```python
from build123d import *
from build123d.topology import SkipClean

# Parameters (mm, degrees)
BOSS_EXTRUDE1_DEPTH = 1.5
SKETCH3_R           = 3.75
CUT_EXTRUDE1_DEPTH  = 0.9
SKETCH4_R           = 2.2
CUT_EXTRUDE2_DEPTH  = 0.9
SKETCH5_R           = 1.5
CUT_EXTRUDE3_DEPTH  = 6
CUT_EXTRUDE4_DEPTH  = 0.3


with BuildPart() as part:
    # Sketch1 → Boss-Extrude1 (new body)
    with BuildSketch(Plane(origin=(0, 0, 0), x_dir=(1, 0, 0), z_dir=(0, 1, 0))):
        Polygon((-13.430051813, 17.5), (-13.430051813, 0), (-11.430051813, 0), (-11.430051813, -2.5), (8.569948187, -2.5), (8.569948187, 0), (10.569948187, 0), (10.569948187, 17.5), align=None)
    extrude(amount=BOSS_EXTRUDE1_DEPTH)

    # Sketch3 → Cut-Extrude1 (cut)
    with BuildSketch(Plane.XZ):
        with Locations(Location((-1.430051813, -7.5, 0), (0, 0, 270))):
            Circle(SKETCH3_R)
    extrude(amount=-CUT_EXTRUDE1_DEPTH, mode=Mode.SUBTRACT)

    # Sketch4 → Cut-Extrude2 (cut)
    with BuildSketch(Plane.XZ.offset(-0.9)):
        with Locations(Location((-1.430051813, -7.5, 0), (0, 0, 270))):
            Circle(SKETCH4_R)
    extrude(amount=-CUT_EXTRUDE2_DEPTH, mode=Mode.SUBTRACT)

    # Sketch5 → Cut-Extrude3 (cut)
    with BuildSketch(Plane.XZ):
        with Locations(Location((-8.430051813, -13.5, 0), (0, 0, 270))):
            Circle(SKETCH5_R)
        with Locations(Location((5.569948187, -13.5, 0), (0, 0, 270))):
            Circle(SKETCH5_R)
    extrude(amount=-CUT_EXTRUDE3_DEPTH, mode=Mode.SUBTRACT)

    # Sketch6 → Cut-Extrude4 (cut)
    with SkipClean():  # the faces are left unmerged after this step: merging them gives an invalid solid
        with BuildSketch(Plane.XZ.offset(-0.9)):
            with BuildLine():
                Line((1.606805114, -9.7), (-4.466908741, -9.7))
                ThreePointArc((-4.466908741, -9.7), (-5.180051813, -7.5), (-4.466908741, -5.3))
                Line((-4.466908741, -5.3), (1.606805114, -5.3))
                ThreePointArc((1.606805114, -5.3), (2.319948187, -7.5), (1.606805114, -9.7))
            make_face()
        extrude(amount=-CUT_EXTRUDE4_DEPTH, mode=Mode.SUBTRACT)


solid = part.part
```
The model under review builds one solid part; all positions refer to its coordinate system, in mm. A direction names the side the tool comes from. Round coordinates to 2 decimals unless told otherwise and drop trailing zeros. Loops run counter-clockwise (first coordinate to the right, second up) from the corner with the lowest first, then second, coordinate; pieces in that order, holes last. Notation, with made-up numbers: (9, 51.25) -> (53, 51.25) arc R24 ccw to (53, 63.25) -> close; hole circle Ø2 at (-31, 73). An arc over 180 degrees is marked (long way). Answer as a JSON object with one key per item and string values. Group by question number.
1) Mouldability with a two-part tool opening along X and no side actions: class faces 5 (the face through (-2, 0, -12)), 6 (the face through (-4, 1.2, -7)), 7 (the face through (8.57, 1, 1)) as released by +X, released by -X, zero draft, split by the parting line, or undercut.
2) For line 1 (X direction, y = 0.7, z = -13.5); line 2 (X direction, y = 1.35, z = -7.5); line 3 (Z direction, x = -4.5, y = 0.3), list the stretches that pass through material, from the lowest coordinate up. Write a range as [from, to].
3) For faces 1 (the face through (10, 1, 0)), 2 (the face through (-1, 0.9, -5)), 3 (the face through (-12, 1, 0)), 4 (the face through (5.6, 0.7, -12)), list the 3-axis set-ups (+Z, -Z, +X, -X, +Y, -Y) from which the entire face can be reached by the end or side of a thin tool; tool diameter is ignored.
4) We need section B-B on x = -1. Write out the cut boundary in (y, z).
5) For pin 1 Ø1.1 at (x, z) = (0.5, -8) entering from -Y; pin 2 Ø4 at (x, z) = (-1.43, -7.5) entering from -Y; pin 3 Ø0.8 at (y, z) = (1, 0.5) entering from +X; pin 4 Ø0.8 at (x, z) = (-2.5, -4.5) entering from -Y, all flat-tipped, find the tip position at first contact; note any pin that passes through.
6) We need section A-A on z = -13.5. Write out the cut boundary in (x, y).
Result set:
{
 "1": {"face 5": "zero draft", "face 6": "undercut", "face 7": "released by +X"},
 "2": {"line 1": "[-13.43, -9.93], [-6.93, 4.07], [7.07, 10.57]", "line 2": "[-13.43, -3.63], [0.77, 10.57]", "line 3": "[-17.5, -9.65], [-5.35, 2.5]"},
 "3": {"face 1": "+Z, +X, +Y, -Y", "face 2": "-Y", "face 3": "+Z, -X, +Y, -Y", "face 4": "+Y, -Y"},
 "4": {"outline": "(0, -17.5) -> (1.5, -17.5) -> (1.5, -9.66) -> (1.2, -9.66) -> (1.2, -9.7) -> (0.9, -9.7) -> (0.9, -11.23) -> (0, -11.23) -> close; (0, -3.77) -> (0.9, -3.77) -> (0.9, -5.3) -> (1.2, -5.3) -> (1.2, -5.34) -> (1.5, -5.34) -> (1.5, 2.5) -> (0, 2.5) -> close"},
 "5": {"pin 1": "y = 1.2", "pin 2": "through", "pin 3": "x = 8.57", "pin 4": "y = 0.9"},
 "6": {"outline": "(-13.43, 0) -> (-9.93, 0) -> (-9.93, 1.5) -> (-13.43, 1.5) -> close; (-6.93, 0) -> (4.07, 0) -> (4.07, 1.5) -> (-6.93, 1.5) -> close; (7.07, 0) -> (10.57, 0) -> (10.57, 1.5) -> (7.07, 1.5) -> close"}
}
